Geometry: final body of the model. Coordinates: model frame, mm. A direction names the side the tool comes from. Round coordinates to 2 decimals unless told otherwise and drop trailing zeros. Order: outer loops, then holes, each group sorted by start corner. A loop starts at its lowest first (then second) coordinate and runs counter-clockwise, first axis right, second up. Notation, with made-up numbers: M -32.5,77.5 L -27.5,77.5 A22 ccw -27.5,89.5 Z; hole C 69.25,-8 d3. An arc over 180 degrees is marked long. Return JSON: item names as keys, results as strings. Group by question number.
Q1. Mould query, pull axis Y, two halves, no side actions, for faces 1 (the face through (39, -8, 1)), 2 (the face through (7, -2.5, 1)), 3 (the face through (-4.417, 0.863, 0.986)). Classes: released by +Y, released by -Y, zero draft, split by the parting line, or undercut.
Q2. Access query for faces 4 (the face through (20, -2, 2)), 5 (the face through (42, 0, 1)), 6 (the face through (7, -4.5, 1)), 7 (the face through (0.924, -6.129, 0.986)), 8 (the face through (41, -2.5, 1)). Directions: +Z, -Z, +X, -X, +Y, -Y. A direction counts if a zero-diameter tool reaches every point of the face in a straight line with its end or side. Return the directions, or none.
Q3. Cut plane C-C on x = 32.5. Output: boundary loops of the cut face in (y, z).
Q4. Ray query, probe 1 along Y at (x, z) = (10, 0.4); probe 2 along Y at (x, z) = (8.5, 1.45); probe 3 along Y at (x, z) = (40, 1.4). Return the intervals inside material, ascending.
Q5. Cut plane B-B on z = 0.6. Count the separate pieces of the cut face and the enclosed holes in it, and give its area (3 significant figures).
Q6. Cut plane A-A on x = 11. Output: boundary loops of the cut face in (y, z), and give its area (3 significant figures).
Q7. Contact query for flat-ended pins moving along their axis: pin 1 (0.6 mm diameter, centred on y = -3.5, z = 1, fed in from +X); pin 2 (1 mm diameter, centred on y = 8.5, z = 0, fed in from -X); pin 3 (0.6 mm diameter, centred on x = 9, z = 0.5, fed in from +Y). Output: stop coordinate, or through.
```python
from build123d import *

# Parameters (mm, degrees)
SKETCH1_R           = 1.75
SKETCH1_W           = 6
SKETCH1_H           = 2
BOSS_EXTRUDE1_DEPTH = 2


with BuildPart() as part:
    # Sketch1 → Boss-Extrude1 (new body)
    with BuildSketch(Plane.XY):
        with BuildLine():
            Line((4.690618402, 5.725955542), (2.844900384, 4.433569872))
            ThreePointArc((2.844900384, 4.433569872), (2.189215725, 4.176328188), (1.488401797, 4.246723454))
            ThreePointArc((1.488401797, 4.246723454), (-4.436229003, 0.754898821), (0, -4.5))
            Line((0, -4.5), (0, -5.281879049))
            Line((0, -5.281879049), (1.875, -7))
            Line((1.875, -7), (13.125, -7))
            Line((13.125, -7), (14.761962752, -5.5))
            Line((14.761962752, -5.5), (31.536424497, -5.5))
            Line((31.536424497, -5.5), (34.26469575, -8))
            Line((34.26469575, -8), (43.158691499, -8))
            Line((43.158691499, -8), (44.25, -7))
            Line((44.25, -7), (44.25, -4.5))
            Line((44.25, -4.5), (38.25, -4.5))
            Line((38.25, -4.5), (38.25, -2.5))
            Line((38.25, -2.5), (44.25, -2.5))
            Line((44.25, -2.5), (44.25, 0))
            Line((44.25, 0), (39.069245955, 0))
            ThreePointArc((39.069245955, 0), (37.504901305, 0.123116594), (35.979076012, 0.489434837))
            Line((35.979076012, 0.489434837), (15.082734658, 7.279067722))
            ThreePointArc((15.082734658, 7.279067722), (14.482691436, 7.647908864), (14.117151245, 8.249968682))
            ThreePointArc((14.117151245, 8.249968682), (9.164682181, 11.333488621), (5.330146444, 6.936742015))
            ThreePointArc((5.330146444, 6.936742015), (5.156603875, 6.254115739), (4.690618402, 5.725955542))
        make_face()
        Circle(SKETCH1_R, mode=Mode.SUBTRACT)
        with Locations((9.829824531, 6.882917236)):
            Circle(SKETCH1_R, mode=Mode.SUBTRACT)
        with Locations((7.5, -3.5)):
            Rectangle(SKETCH1_W, SKETCH1_H, mode=Mode.SUBTRACT)
        with BuildLine():
            Line((13.84666668, 3.474841657), (26.75576114, -0.719577393))
            ThreePointArc((26.75576114, -0.719577393), (27.027229678, -1.162573786), (26.632154342, -1.5))
            Line((26.632154342, -1.5), (14.761962752, -1.5))
            Line((14.761962752, -1.5), (13.125, 0))
            Line((13.125, 0), (4.5, 0))
            ThreePointArc((4.5, 0), (4.487297154, 0.337882015), (4.449260331, 0.673856446))
            Line((4.449260331, 0.673856446), (6.984924148, 2.449347365))
            ThreePointArc((6.984924148, 2.449347365), (7.640608806, 2.706589049), (8.341422735, 2.636193783))
            ThreePointArc((8.341422735, 2.636193783), (10.494966882, 2.432345851), (12.494812024, 3.256921971))
            ThreePointArc((12.494812024, 3.256921971), (13.144422133, 3.529139461), (13.84666668, 3.474841657))
        make_face(mode=Mode.SUBTRACT)
    extrude(amount=BOSS_EXTRUDE1_DEPTH)


solid = part.part
```
Result sheet:
{
 "1": {"face 1": "released by -Y", "face 2": "undercut", "face 3": "split by the parting line"},
 "2": {"face 4": "+Z, +X, -X, +Y, -Y", "face 5": "+Z, -Z, +X, +Y", "face 6": "+Z, -Z", "face 7": "+Z, -Z, -X, -Y", "face 8": "+Z, -Z, +X"},
 "3": {"outline": "M -6.38,0 L 1.62,0 L 1.62,2 L -6.38,2 Z"},
 "4": {"probe 1": "y = -7 to -4.5, -2.5 to 0, 2.39 to 5.14, 8.62 to 11.38", "probe 2": "y = -7 to -4.5, -2.5 to 0, 2.58 to 5.75, 8.02 to 11.18", "probe 3": "y = -8 to -4.5, -2.5 to 0"},
 "5": {"separate pieces": "1", "enclosed holes": "4", "area": "426 mm²"},
 "6": {"outline": "M -7,0 L 0,0 L 0,2 L -7,2 Z; M 2.54,0 L 5.58,0 L 5.58,2 L 2.54,2 Z; M 8.18,0 L 11.23,0 L 11.23,2 L 8.18,2 Z", "area": "26.2 mm²"},
 "7": {"pin 1": "stops at x = 38.25", "pin 2": "stops at x = 5.47", "pin 3": "stops at y = 11.35"}
}
